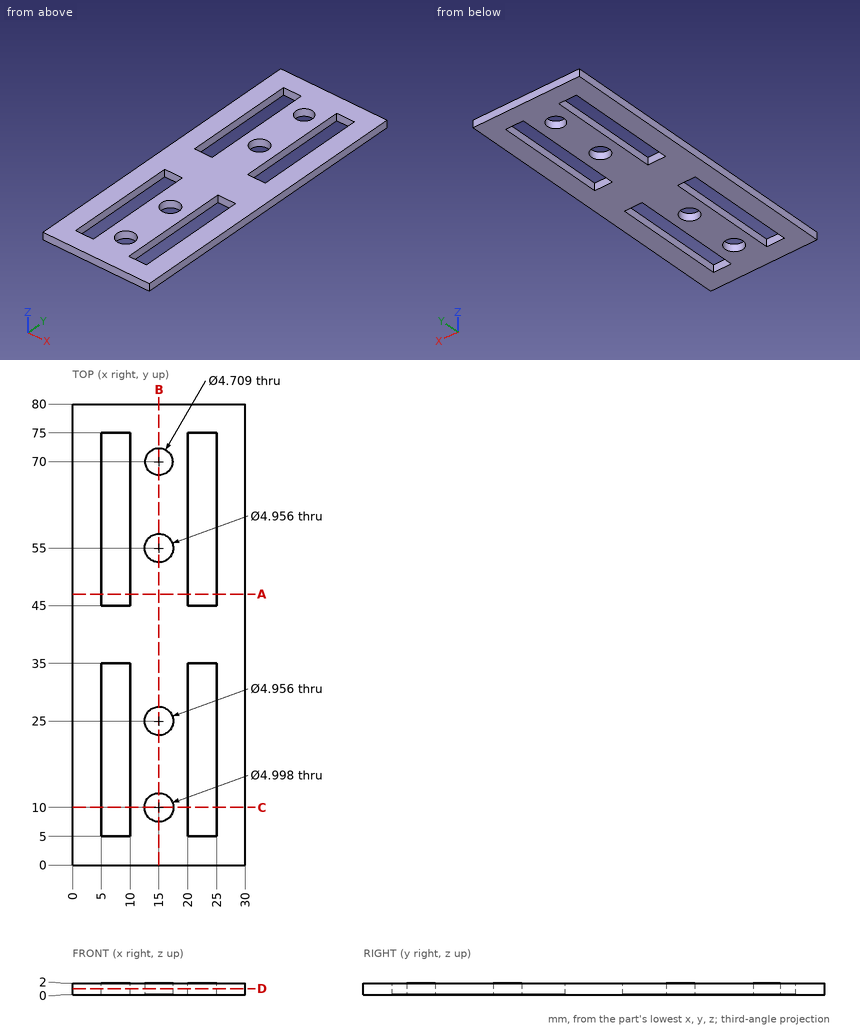
Drawing for the job (mm, zero at the part's lowest x, y, z). Coordinates: 2 decimals unless noted, no trailing zeros. Order: outer loops, then holes, each group sorted by start corner. A loop starts at its lowest first (then second) coordinate and runs counter-clockwise, first axis right, second up. Notation, with made-up numbers: (66.25, 16.25) -> (124.25, 16.25) arc R21 ccw to (124.25, 31.25) -> close; hole circle Ø8 at (-32.5, -29.75). An arc over 180 degrees is marked (long way). Answer in a Markdown table with one row per item.
1) Drill centre lines: line 1 (X direction, y = 51.5, z = 0.5); line 2 (Y direction, x = 15, z = 0.9) (1 decimal); line 3 (Y direction, x = 7.5, z = 1.4). Where is each one in solid material? Low to high.
Check values:
| item | result |
|---|---|
| line 1 | 0 to 5, 10 to 20, 25 to 30 |
| line 2 | 0 to 7.5, 12.5 to 22.5, 27.5 to 52.5, 57.5 to 67.6, 72.4 to 80 |
| line 3 | 0 to 5, 35 to 45, 75 to 80 |
2) Band-saw the part on C-C (y = 10). List the corners of the cut face in (x, z).
Check values:
| item | result |
|---|---|
| outline | (0, 0) -> (5, 0) -> (5, 2) -> (0, 2) -> close; (10, 0) -> (12.5, 0) -> (12.5, 2) -> (10, 2) -> close; (17.5, 0) -> (20, 0) -> (20, 2) -> (17.5, 2) -> close; (25, 0) -> (30, 0) -> (30, 2) -> (25, 2) -> close |
3) Band-saw the part on D-D (z = 1.05). Give the number of separate pieces and of enclosed holes in the cut face, and give its area (3 significant figures).
Check values:
| item | result |
|---|---|
| separate pieces | 1 |
| enclosed holes | 8 |
| area | 1,720 mm2 |
4) Band-saw the part on B-B (x = 15). List the corners of the cut face in (y, z) (1 decimal), and give its area (3 significant figures).
Check values:
| item | result |
|---|---|
| outline | (0, 0) -> (7.5, 0) -> (7.5, 2) -> (0, 2) -> close; (12.5, 0) -> (22.5, 0) -> (22.5, 2) -> (12.5, 2) -> close; (27.5, 0) -> (52.5, 0) -> (52.5, 2) -> (27.5, 2) -> close; (57.5, 0) -> (67.6, 0) -> (67.6, 2) -> (57.5, 2) -> close; (72.4, 0) -> (80, 0) -> (80, 2) -> (72.4, 2) -> close |
| area | 121 mm2 |
5) Band-saw the part on A-A (y = 47). List the corners of the cut face in (x, z), and give its area (3 significant figures).
Check values:
| item | result |
|---|---|
| outline | (0, 0) -> (5, 0) -> (5, 2) -> (0, 2) -> close; (10, 0) -> (20, 0) -> (20, 2) -> (10, 2) -> close; (25, 0) -> (30, 0) -> (30, 2) -> (25, 2) -> close |
| area | 40.0 mm2 |
